For this review, take the finished solid that the model builds, in its own axes (mm). Round coordinates to 2 decimals unless told otherwise and drop trailing zeros. Loops run counter-clockwise (first coordinate to the right, second up) from the corner with the lowest first, then second, coordinate; pieces in that order, holes last. Notation, with made-up numbers: (-1.5, 41) -> (6.5, 41) arc R21 ccw to (6.5, 45) -> close; hole circle Ø6 at (65.25, 51). An arc over 180 degrees is marked (long way). Write each question's results on one line, items separated by ' | '.
```python
from build123d import *

# Parameters (mm, degrees)
F0_W     = 347.3
F0_H     = 51.58
F0_R     = 3.3
F0_R_2   = 5
F1_DEPTH = 6.35
F3_D     = 6.6
F4_R     = 1.4
F5_DEPTH = 6.351


# Not quite as in the source:
# - a feature names something its author has since deleted; it is built from what else it names


with BuildPart() as f1:
    # F0 (on Top) → F1 (new body)
    with BuildSketch(Plane.XY):
        Rectangle(F0_W, F0_H)
        with Locations((-125, 0)):
            Circle(F0_R, mode=Mode.SUBTRACT)
        Circle(F0_R_2, mode=Mode.SUBTRACT)
        with Locations((125, 0)):
            Circle(F0_R, mode=Mode.SUBTRACT)
    extrude(amount=F1_DEPTH)

    # F3 (through all)
    with Locations(Plane(origin=(0, 0, 0), x_dir=(1, 0, 0), z_dir=(0, 0, -1))):
        with Locations((-162.023125, 12.895), (-162.023125, -12.895), (162.023125, -12.895), (162.023125, 12.895)):
            Hole(F3_D / 2)

    # F4 (on face) → F5 (cut, through all)
    with BuildSketch(Plane.XY.offset(6.35)):
        with Locations((-125, 8.78)):
            Circle(F4_R)
        with Locations((-132.6037030452, -4.39)):
            Circle(F4_R)
        with Locations((-117.3962969548, -4.39)):
            Circle(F4_R)
        with Locations((125, 8.78)):
            Circle(F4_R)
        with Locations((132.6037030452, -4.39)):
            Circle(F4_R)
        with Locations((117.3962969548, -4.39)):
            Circle(F4_R)
    extrude(amount=-F5_DEPTH, mode=Mode.SUBTRACT)


solid = f1.part
```
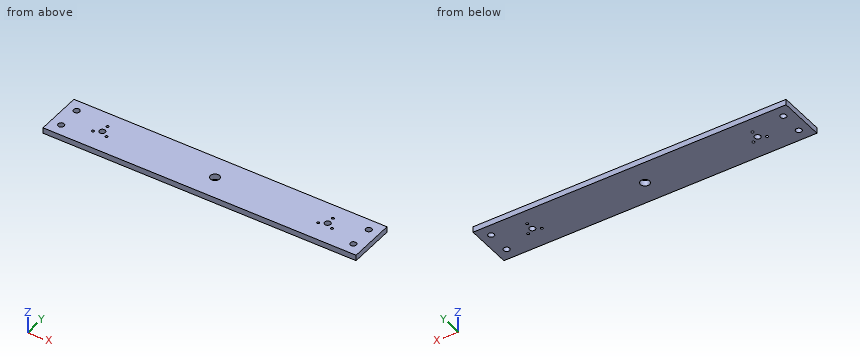
1. To check wall thickness, follow probe 1 along Y at (x, z) = (-125, 4.25); probe 2 along X at (y, z) = (-4.5, 2.25); probe 3 along X at (y, z) = (10, 5.5). State the ranges of each line that lie inside material, in increasing order.
Values found:
probe 1: y = -25.79 to -3.3, 3.3 to 7.38, 10.18 to 25.79 | probe 2: x = -173.65 to -134, -131.21 to -118.79, -116 to -2.18, 2.18 to 116, 118.79 to 131.21, 134 to 173.65 | probe 3: x = -173.65 to -163.61, -160.44 to -125.69, -124.31 to 124.31, 125.69 to 160.44, 163.61 to 173.65
2. Consider section C-C (z = 1). Give the number of separate pieces and of enclosed holes in the cut face, plus the area to 3 significant figures.
Values found:
separate pieces: 1 | enclosed holes: 13 | area: 17,600 mm2
3. Consider section A-A (x = 0). State the section outline as (y, z) points, plus the area to 3 significant figures.
Values found:
outline: (-25.79, 0) -> (-5, 0) -> (-5, 6.35) -> (-25.79, 6.35) -> close; (5, 0) -> (25.79, 0) -> (25.79, 6.35) -> (5, 6.35) -> close | area: 264 mm2
4. For pin 1 (4 mm diameter, centred on x = -125, y = 0, fed in from -Z), flat-tipped, find the tip position at first contact; note if it passes through.
Values found:
pin 1: passes through
5. Consider section B-B (y = 0). State the section outline as (x, z) points, plus the area to 3 significant figures.
Values found:
outline: (-173.65, 0) -> (-128.3, 0) -> (-128.3, 6.35) -> (-173.65, 6.35) -> close; (-121.7, 0) -> (-5, 0) -> (-5, 6.35) -> (-121.7, 6.35) -> close; (5, 0) -> (121.7, 0) -> (121.7, 6.35) -> (5, 6.35) -> close; (128.3, 0) -> (173.65, 0) -> (173.65, 6.35) -> (128.3, 6.35) -> close | area: 2,060 mm2
